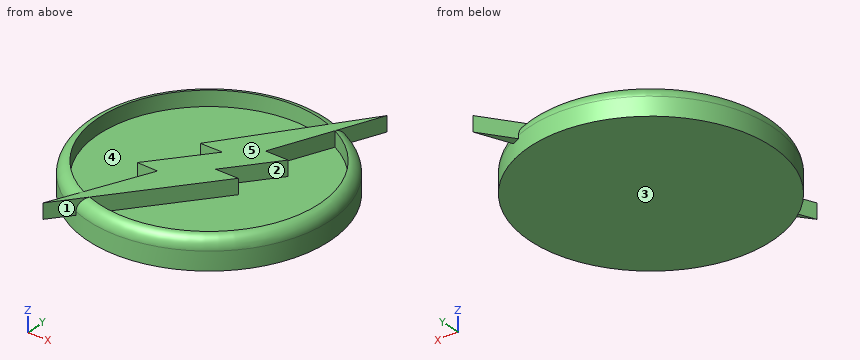
```python
from build123d import *

# Parameters (mm, degrees)
F0_R     = 46.303997109
F1_DEPTH = 6.35
F0_R_2   = 50.7773250867
F2_DEPTH = 12.7
F5_DEPTH = 6.35


# Not quite as in the source:
# - a fillet or chamfer that OpenCascade refuses, or shapes differently, is made with other operations: its cross-section is extruded or revolved along the edge and cut away or added


with BuildPart() as f1:
    # F0 (on Top) → F1 (new body)
    with BuildSketch(Plane.XY):
        Circle(F0_R)
    extrude(amount=F1_DEPTH)

    # F0 (on Top) → F2 (join)
    with BuildSketch(Plane.XY):
        Circle(F0_R_2)
        Circle(F0_R, mode=Mode.SUBTRACT)
    extrude(amount=F2_DEPTH)

    # F3: fillet of radius 5.08 on 1 edges, made by hand

    # F3_s1 → F3_t2 (revolve, cut)
    with BuildSketch(Plane.XZ):
        with BuildLine():
            ThreePointArc((50.7777250867, 7.6554991612), (49.4982109042, 11.0268790536), (46.3040449454, 12.7003971293))
            Line((46.3040449454, 12.7003971293), (46.3648134998, 13.2048869261))
            ThreePointArc((46.3648134998, 13.2048869261), (48.540685016, 13.2081365685), (50.7773250867, 13.2081365685))
            Line((50.7773250867, 13.2081365685), (51.2854616553, 12.7))
            ThreePointArc((51.2854616553, 12.7), (51.2854616553, 10.1777495806), (51.2858616553, 7.6554991612))
            Line((51.2858616553, 7.6554991612), (50.7777250867, 7.6554991612))
        make_face()
    revolve(axis=Axis((0, 0, 12.7), (0, 0, 1)), mode=Mode.SUBTRACT)

    # F4 (on face) → F5 (join)
    with BuildSketch(Plane.XY.offset(6.35)):
        Polygon((-9.3244733289, -15.8572378275), (-26.3735784938, -55.8334334653), (14.7386826575, -3.0078946147), (5.1134219393, -3.0078946147), (20.4086864271, 16.6451374931), (10.8284205198, 16.6451374931), (28.2742083073, 59.8571076989), (-9.3244733289, 7.2189471684), (0, 7.2189471684), (-18.0473700166, -15.6410522759), align=None)
    extrude(amount=F5_DEPTH)


solid = f1.part
```
Part model, mm, in its own coordinate system. Face numbers are marked on the shaded views. A direction names the side the tool comes from. Round coordinates to 2 decimals unless told otherwise and drop trailing zeros. Loops run counter-clockwise (first coordinate to the right, second up) from the corner with the lowest first, then second, coordinate; pieces in that order, holes last.
Item 1: Drop flat-ended pins along their axis: P1, Ø3, axis at x = 9.5, z = 9, coming from the +Y side; P2, Ø4, axis at x = -37, z = 3.5, coming from the -Y side; P3, Ø4, axis at x = -11.5, y = 13.5, coming from the +Z side. Give the stop position or say it passes through.
Item 2: Drill centre lines: line 1 (X direction, y = 10.5, z = 11.75); line 2 (X direction, y = -8, z = 9.75); line 3 (Y direction, x = 4, z = 9.5). Where is each one in solid material? Low to high.
Item 3: Cut at C-C, the plane z = 2.5. Give the cut face in (x, y).
Item 4: Mould opens along Y. For the marked faces 1, 2 and 3 say: +Y half, -Y half, draft (parallel to the pull), parting line (faces both ways), or undercut.
Item 5: 3-axis set-ups, long thin cutter, end or side, ignore diameter. For the marked faces 4 and 5: which of +Z, -Z, +X, -X, +Y, -Y reach the whole face in a straight line?
A:
1. P1: stops at y = 50.08
1. P2: stops at y = -36.79
1. P3: stops at z = 6.35
2. line 1: x = -47.56 to -45.1, -6.98 to 15.63, 45.1 to 47.56
2. line 2: x = -49.69 to -45.61, -12.01 to 10.85, 45.61 to 49.69
2. line 3: y = -50.27 to -46.13, -16.81 to 25.87, 46.13 to 50.27
3. outline: circle Ø101.55 at (0, 0)
4. face 1: -Y half
4. face 2: undercut
4. face 3: draft
5. face 4: +Z
5. face 5: +Z, +X, -X, +Y, -Y
